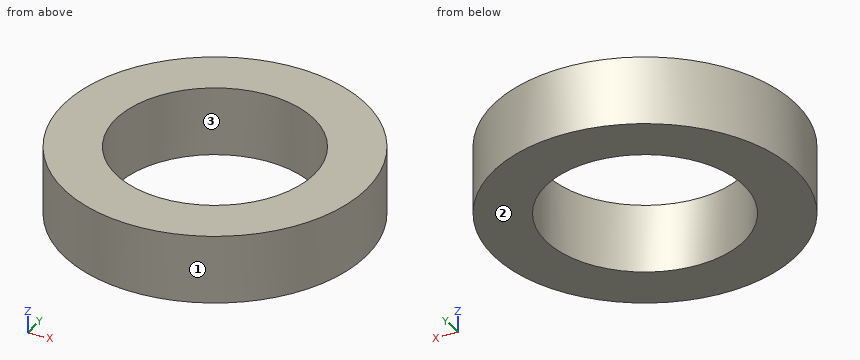
from build123d import *

# Parameters (mm, degrees)
F_0172_CYLINDER_SKETCH_R = 5.5
F_0172_CYLINDER_DEPTH    = 2.5
F_0173_CYLINDER_SKETCH_R = 3.6
F_0173_CYLINDER_DEPTH    = 5


with BuildPart() as part:
    # 0172_cylinder_Sketch → 0172_cylinder (new body)
    with BuildSketch(Plane.XY):
        Circle(F_0172_CYLINDER_SKETCH_R)
    extrude(amount=F_0172_CYLINDER_DEPTH)


with BuildPart() as body_2:
    # 0173_cylinder_Sketch → 0173_cylinder (new body)
    with BuildSketch(Plane.XY):
        Circle(F_0173_CYLINDER_SKETCH_R)
    extrude(amount=F_0173_CYLINDER_DEPTH)


with BuildPart() as body_2_1:
    # 0173_cylinder_Translate: moved
    add(body_2.part.moved(Location((0, 0, -2.5))))


with BuildPart() as part_1:
    add(part.part)

    # 0174_sub: cut body 2
    add(body_2_1.part, mode=Mode.SUBTRACT)


solid = part_1.part
Can you work these out from the model? Positions are in its coordinate system, mm. Face numbers are marked on the shaded views. Round coordinates to 2 decimals unless told otherwise and drop trailing zeros. Write each loop counter-clockwise with the first axis right and the second up, starting at its lowest first coordinate (ties: lowest second). Pieces come first, ordered by that corner, then holes. Notation, with made-up numbers: (-2, 48.25) - (15, 48.25) arc R20 ccw to (15, 54.25) - close; hole circle Ø7 at (65, 22.5). An arc over 180 degrees is marked (long way). Write each question's results on one line, items separated by ' | '. Start each with the question number.
1) Suppose I cut it at A-A (y = 0). List the corners of the cut face in (x, z) for me, and give its area (3 significant figures).
2) Suppose I cut it at D-D (x = -3.75). List the corners of the cut face in (y, z) for me, and give its area (3 significant figures).
3) Suppose I cut it at C-C (z = 1.25). List the corners of the cut face in (x, y) for me.
4) We'd pull the mould along Y, two halves only. Please class the marked faces 1, 2 and 3: released by +Y, released by -Y, zero draft, split by the parting line, or undercut.
5) Please list where these lines run through material, in increasing order: line 1 (Y direction, x = 0, z = 0.7); line 2 (Y direction, x = 1.5, z = 0.2); line 3 (X direction, y = 2.5, z = 1.3).
Here are the results:
1) outline: (-5.5, 0) - (-3.6, 0) - (-3.6, 2.5) - (-5.5, 2.5) - close; (3.6, 0) - (5.5, 0) - (5.5, 2.5) - (3.6, 2.5) - close | area: 9.50 mm2
2) outline: (-4.02, 0) - (4.02, 0) - (4.02, 2.5) - (-4.02, 2.5) - close | area: 20.1 mm2
3) outline: circle Ø11 at (0, 0); hole circle Ø7.2 at (0, 0)
4) face 1: split by the parting line | face 2: zero draft | face 3: undercut
5) line 1: y = -5.5 to -3.6, 3.6 to 5.5 | line 2: y = -5.29 to -3.27, 3.27 to 5.29 | line 3: x = -4.9 to -2.59, 2.59 to 4.9
